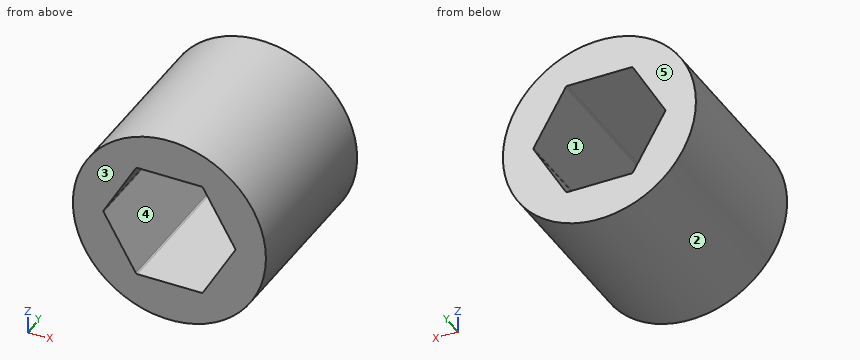
```python
from build123d import *

# Parameters (mm, degrees)
SKETCH1_R           = 11.1125
BOSS_EXTRUDE1_DEPTH = 20.447
FILLET1_R           = 0.2


with BuildPart() as part:
    # Sketch1 → Boss-Extrude1 (new body)
    with BuildSketch(Plane(origin=(0, 0, 0), x_dir=(1, 0, 0), z_dir=(0, 1, 0))):
        Circle(SKETCH1_R)
        Polygon((7.625642355, 0), (3.812821178, 6.604), (-3.812821178, 6.604), (-7.625642355, 0), (-3.812821178, -6.604), (3.812821178, -6.604), align=None, mode=Mode.SUBTRACT)
    extrude(amount=BOSS_EXTRUDE1_DEPTH)

    # Fillet1
    fillet1_edges = [part.edges().sort_by_distance(p)[0] for p in [
        (7.625642355, 10.2235, 0),
        (3.812821178, 10.2235, -6.604),
        (-3.812821178, 10.2235, -6.604),
        (-7.625642355, 10.2235, 0),
        (-3.812821178, 10.2235, 6.604),
        (3.812821178, 10.2235, 6.604),
    ]]
    fillet(fillet1_edges, radius=FILLET1_R)


solid = part.part
```
Can you work these out from the model? Positions are in its coordinate system, mm. Face numbers are marked on the shaded views. A direction names the side the tool comes from. Give positions to 0.01 mm unless a question says otherwise; leave off trailing zeros. Loops run counter-clockwise (first coordinate to the right, second up) from the corner with the lowest first, then second, coordinate; pieces in that order, holes last. Notation, with made-up numbers: M 35,6 L 69,6 A36 ccw 69,42 Z; hole C 13,50.25 d9. An arc over 180 degrees is marked long. One line per item, written item: value.
(1) Suppose I cut it at D-D on z = 9.25. List the corners of the cut face in (x, y) for me, plus the area to 3 significant figures.
Returned:
outline: M -6.16,0 L 6.16,0 L 6.16,20.45 L -6.16,20.45 Z
area: 252 mm^2
(2) I need wall thicknesses on line 1 (Z direction, x = -0.5, y = 3.5); line 2 (Z direction, x = 7, y = 11.25); line 3 (X direction, y = 1.5, z = 4.5). Which ranges of each line are inside material? Lowest first, please.
Returned:
line 1: -11.1 to -6.6, 6.6 to 11.1
line 2: -8.63 to -1.08, 1.08 to 8.63
line 3: -10.16 to -5.03, 5.03 to 10.16
(3) Will these pins go through, and if not, where does the flat tip stop? pin 1 (1 mm diameter, centred on x = 1.5, y = 2, fed in from +Z); pin 2 (4 mm diameter, centred on y = 4.5, z = -6.5, fed in from +X); pin 3 (5 mm diameter, centred on y = 13, z = -5, fed in from -X).
Returned:
pin 1: z = 11.07
pin 2: x = 10.16
pin 3: x = -10.83
(4) Suppose I cut it at C-C on z = 2. List the corners of the cut face in (x, y) for me.
Returned:
outline: M -10.93,0 L -6.47,0 L -6.47,20.45 L -10.93,20.45 Z; M 6.47,0 L 10.93,0 L 10.93,20.45 L 6.47,20.45 Z
(5) Which directions (+Z, -Z, +X, -X, +Y, -Y) give clear straight access to the entire face, cutting with the end or side of a thin tool? Please do the marked faces 4 and 5.
Returned:
face 4: +Y, -Y
face 5: +Z, -Z, +X, -X, +Y
(6) We'd pull the mould along Z, two halves only. Please class the marked faces 1, 2 and 3: released by +Z, released by -Z, zero draft, split by the parting line, or undercut.
Returned:
face 1: undercut
face 2: split by the parting line
face 3: zero draft
(7) Suppose I cut it at B-B on x = 0. List the corners of the cut face in (y, z) for me.
Returned:
outline: M 0,-11.11 L 20.45,-11.11 L 20.45,-6.6 L 0,-6.6 Z; M 0,6.6 L 20.45,6.6 L 20.45,11.11 L 0,11.11 Z
